CAD build for the part. Positions are in the model's coordinates, mm. A direction names the side the tool comes from. Coordinates: 2 decimals unless noted, no trailing zeros. Write each loop counter-clockwise with the first axis right and the second up, starting at its lowest first coordinate (ties: lowest second). Pieces come first, ordered by that corner, then holes. Notation, with made-up numbers: (-6.5, -6.75) -> (23.5, -6.75) arc R10 ccw to (23.5, 3.25) -> close; hole circle Ø1 at (72.25, 59.5). An arc over 180 degrees is marked (long way). Answer as CSV lines item,"result". Start each with the question number.
```python
from build123d import *

# Parameters (mm, degrees)
ESQUISSE1_R             = 5.3
BOSS_EXTRU_1_DEPTH      = 3
ESQUISSE2_R             = 4.239698474
BOSS_EXTRU_2_DEPTH      = 5
ESQUISSE3_R             = 1.75
ENL_V_MAT_EXTRU_1_DEPTH = 64.373180447


with BuildPart() as part:
    # Esquisse1 → Boss.-Extru.1 (new body)
    with BuildSketch(Plane.XY):
        with BuildLine():
            Line((0, 10), (-59.6, 10))
            Line((-59.6, 10), (-59.6, -10))
            Line((-59.6, -10), (0, -10))
            ThreePointArc((0, -10), (10, 0), (0, 10))
        make_face()
        Circle(ESQUISSE1_R, mode=Mode.SUBTRACT)
    extrude(amount=BOSS_EXTRU_1_DEPTH)

    # Esquisse2 → Boss.-Extru.2 (add)
    with BuildSketch(Plane.XY.offset(3)):
        with BuildLine():
            Line((-59.6, 10), (-59.6, -10))
            Line((-59.6, -10), (0, -10))
            ThreePointArc((0, -10), (10, 0), (0, 10))
            Line((0, 10), (-59.6, 10))
        make_face()
        with Locations((-0.060301526, 0)):
            Circle(ESQUISSE2_R, mode=Mode.SUBTRACT)
    extrude(amount=BOSS_EXTRU_2_DEPTH)

    # Esquisse3 → Enlèv. mat.-Extru.1 (cut, through all)
    with BuildSketch(Plane(origin=(0, 10, 0), x_dir=(1, 0, 0), z_dir=(0, 1, 0))):
        with Locations(Location((-54.6, -4, 0), (0, 0, 180))):
            Circle(ESQUISSE3_R)
        with Locations(Location((-44.6, -4, 0), (0, 0, 180))):
            Circle(ESQUISSE3_R)
        with Locations(Location((-34.6, -4, 0), (0, 0, 180))):
            Circle(ESQUISSE3_R)
        with Locations(Location((-24.6, -4, 0), (0, 0, 180))):
            Circle(ESQUISSE3_R)
        with Locations(Location((-14.6, -4, 0), (0, 0, 180))):
            Circle(ESQUISSE3_R)
    extrude(amount=-ENL_V_MAT_EXTRU_1_DEPTH, mode=Mode.SUBTRACT)


solid = part.part
```
1. Mould opens along Z. For faces 3 (the face through (-30, -10, 4)), 4 (the face through (-25, 0, 8)), 5 (the face through (-16.217, 0.14, 3.33)) say: pulls with the +Z half, pulls with the -Z half, needs draft (parallel to the pull), parting line crosses it, or undercut.
2. Flat gauge pin, fed straight in: P1, Ø2, axis at x = -44.6, z = 4, coming from the -Y side. Where does the tip first touch, or does it go through?
3. Tool access for faces 1 (the face through (10, 0, 4)), 2 (the face through (4.896, -2.03, 1.479)): list every direction of +Z, -Z, +X, -X, +Y, -Y with a clear straight run to the whole face (end or side of a thin tool).
4. Cut at D-D (y = -6.5). Give the cut face in (x, z), then the cut area to 3 significant figures.
5. Wall check: line 1 (Z direction, x = -24.5, y = -3.5); line 2 (X direction, y = -2.5, z = 1.5); line 3 (X direction, y = 9, z = 5.5). Give the ranges that are in metal, low to high.
6. Cut at C-C (z = 1.25). Give the cut face in (x, y).
7. Cut at A-A (x = -34.6). Give the cut face in (y, z), then the cut area to 3 significant figures.
8. Cut at B-B (y = 0). Give the cut face in (x, z).
Geometry check:
1,face 3,"needs draft"
1,face 4,"pulls with the +Z half"
1,face 5,"undercut"
2,P1,"through"
3,face 1,"+Z, -Z, +X"
3,face 2,"-Z"
4,outline,"(-59.6, 0) -> (7.6, 0) -> (7.6, 8) -> (-59.6, 8) -> close; hole circle Ø3.5 at (-54.6, 4); hole circle Ø3.5 at (-44.6, 4); hole circle Ø3.5 at (-34.6, 4); hole circle Ø3.5 at (-24.6, 4); hole circle Ø3.5 at (-14.6, 4)"
4,area,"489 mm²"
5,line 1,"0 to 2.25, 5.75 to 8"
5,line 2,"-59.6 to -4.67, 4.67 to 9.68"
5,line 3,"-59.6 to -55.5, -53.7 to -45.5, -43.7 to -35.5, -33.7 to -25.5, -23.7 to -15.5, -13.7 to 4.36"
6,outline,"(-59.6, -10) -> (0, -10) arc R10 ccw to (0, 10) -> (-59.6, 10) -> close; hole circle Ø10.6 at (0, 0)"
7,outline,"(-10, 0) -> (10, 0) -> (10, 2.25) -> (-10, 2.25) -> close; (-10, 5.75) -> (10, 5.75) -> (10, 8) -> (-10, 8) -> close"
7,area,"90.0 mm²"
8,outline,"(-59.6, 0) -> (-5.3, 0) -> (-5.3, 3) -> (-4.3, 3) -> (-4.3, 8) -> (-59.6, 8) -> close; (4.18, 3) -> (5.3, 3) -> (5.3, 0) -> (10, 0) -> (10, 8) -> (4.18, 8) -> close; hole circle Ø3.5 at (-54.6, 4); hole circle Ø3.5 at (-44.6, 4); hole circle Ø3.5 at (-34.6, 4); hole circle Ø3.5 at (-24.6, 4); hole circle Ø3.5 at (-14.6, 4)"
